Could you check a few things on this model? Use its own coordinates, in mm. A direction names the side the tool comes from. Coordinates: 2 decimals unless noted, no trailing zeros. Write each loop counter-clockwise with the first axis right and the second up, starting at its lowest first coordinate (ties: lowest second). Pieces come first, ordered by that corner, then holes. Notation, with made-up numbers: M 63.5,-34.75 L 112.5,-34.75 A16 cw 112.5,-26.75 Z; hole C 44.25,16 d8. An arc over 180 degrees is marked long. Write item = value, one per line.
```python
from build123d import *

# Parameters (mm, degrees)
SKETCH1_R               = 76.2
BOSS_EXTRUDE1_DEPTH     = 6.35
CUT_EXTRUDE3_DEPTH      = 108.95
CUT_EXTRUDE3_DEPTH_BACK = 108.95
SKETCH1_4_R             = 4.7625
SKETCH2_R               = 3.175
CUT_EXTRUDE4_DEPTH      = 3.175


with BuildPart() as part:
    # Sketch1 → Boss-Extrude1 (new body)
    with BuildSketch(Plane.XY):
        Circle(SKETCH1_R)
    extrude(amount=BOSS_EXTRUDE1_DEPTH)

    # Sketch1<4> → Cut-Extrude3 (cut, two sides: drawn at the far end of the back side and taken through both)
    with BuildSketch(Plane.XY.offset(-CUT_EXTRUDE3_DEPTH_BACK)):
        Circle(SKETCH1_4_R)
    extrude(amount=CUT_EXTRUDE3_DEPTH + CUT_EXTRUDE3_DEPTH_BACK, mode=Mode.SUBTRACT)

    # Sketch2 → Cut-Extrude4 (cut)
    with BuildSketch(Plane(origin=(0, 0, 0), x_dir=(-1, 0, 0), z_dir=(0, 0, -1))):
        with Locations((0, 63.5)):
            Circle(SKETCH2_R)
        with Locations((0, -63.5)):
            Circle(SKETCH2_R)
    extrude(amount=-CUT_EXTRUDE4_DEPTH, mode=Mode.SUBTRACT)


solid = part.part
```
Item 1: Imagine slicing it at C-C (z = 2). State how many separate pieces and enclosed holes the cut face has, and give its area (3 significant figures).
Numbers:
separate_pieces = 1
enclosed_holes = 3
area = 18,100 mm²
Item 2: I'm going to push flat-ended pins straight in: P1, Ø1, axis at x = 10.5, z = 4.5, coming from the -Y side; P2, Ø1, axis at x = -48, z = 4.5, coming from the +Y side; P3, Ø1, axis at x = -56.5, z = 4, coming from the -Y side. Where does each tip first touch, or does it pass through?
Numbers:
P1 = -75.54
P2 = 59.58
P3 = -51.68
Item 3: Imagine slicing it at B-B (y = 0). Write out the boundary of the cut face in (x, z), and give its area (3 significant figures).
Numbers:
outline = M -76.2,0 L -4.76,0 L -4.76,6.35 L -76.2,6.35 Z; M 4.76,0 L 76.2,0 L 76.2,6.35 L 4.76,6.35 Z
area = 907 mm²
Item 4: For faces 1 (the face through (16, 1, 0)), 2 (the face through (0, 64, 3.175)), which set-ups out of +Z, -Z, +X, -X, +Y, -Y let a thin tool reach every point of the face, with its end or its side?
Numbers:
face_1 = -Z, +X, -X, +Y, -Y
face_2 = -Z
Item 5: Imagine slicing it at D-D (y = 63.5). Write out the boundary of the cut face in (x, z) (3 decimals), and give its area (3 significant figures).
Numbers:
outline = M -42.121,0 L -3.175,0 L -3.175,3.175 L 3.175,3.175 L 3.175,0 L 42.121,0 L 42.121,6.35 L -42.121,6.35 Z
area = 515 mm²
Item 6: If I drill on line 1 along Y through (x, z) = (0, 1.45) (1 decimal); line 2 along Y through (x, z) = (0, 4); line 3 along Y through (x, z) = (-3.5, 1.75), over which ranges is the centre line in solid material (lowest first)?
Numbers:
line_1 = -76.2 to -66.7, -60.3 to -4.8, 4.8 to 60.3, 66.7 to 76.2
line_2 = -76.2 to -4.76, 4.76 to 76.2
line_3 = -76.12 to -3.23, 3.23 to 76.12
Item 7: If we mould it in two halves opening along Y, with no side actions, what happens to faces 3 (the face through (-1.707, 66.177, 1.565)), 4 (the face through (-60.47, -46.367, 3.131)), 5 (the face through (0, -63, 3.175)), 6 (the face through (16, 1, 6.35))? For each: pulls with the +Y half, pulls with the -Y half, needs draft (parallel to the pull), parting line crosses it, or undercut.
Numbers:
face_3 = undercut
face_4 = parting line crosses it
face_5 = undercut
face_6 = needs draft
